Input: part model. Units: mm. Frame: model coordinates. Face numbers are marked on the shaded views. Round coordinates to 2 decimals unless told otherwise and drop trailing zeros. Order: outer loops, then holes, each group sorted by start corner. A loop starts at its lowest first (then second) coordinate and runs counter-clockwise, first axis right, second up.
Item 1: Cut plane C-C on x = -55. Output: boundary loops of the cut face in (y, z).
Item 2: Cut plane B-B on y = -3. Output: boundary loops of the cut face in (x, z).
Item 3: Mould query, pull axis X, two halves, no side actions, for the marked faces 1, 2 and 3. Classes: released by +X, released by -X, zero draft, split by the parting line, or undercut.
Item 4: Line query: L1, parallel to Z at x = 7, y = 21; L2, parallel to X at y = 21, z = -13; L3, parallel to Z at x = -53, y = 18. Output: solid intervals per line, ascending.
Item 5: First-contact query: pin 1 (12 mm diameter, centred on y = 7.5, z = -9, fed in from +X); pin 2 (3.5 mm diameter, centred on x = -7, z = -47.5, fed in from +Y); pin 3 (1.5 mm diameter, centred on y = -14.5, z = -39.5, fed in from +X); pin 4 (5 mm diameter, centred on x = -86.5, y = 11, fed in from +Z). Flat tips, straight axial feed; report the tip coordinate or a pass-through.
Item 6: Cut plane A-A on z = -30.5. Output: boundary loops of the cut face in (x, y), then the cut area to 3 significant figures.
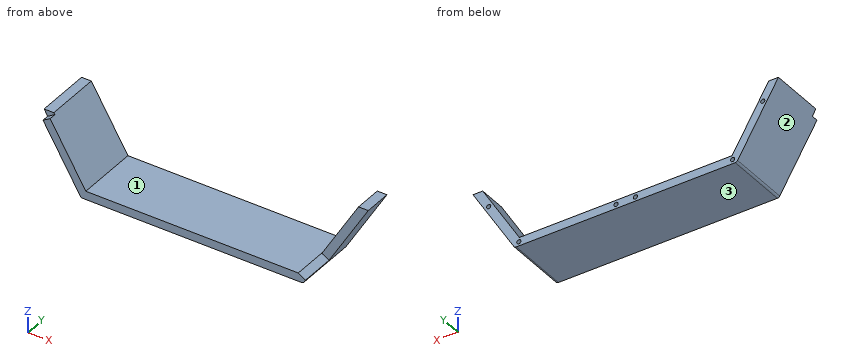
```python
from build123d import *

# Parameters (mm, degrees)
BOSS_EXTRUDE1_DEPTH = 22.5
SKETCH2_R           = 1.5
CUT_EXTRUDE1_DEPTH  = 5
FILLET1_R           = 2
SKETCH4_W           = 55
SKETCH4_H           = 25
CUT_EXTRUDE3_DEPTH  = 10
SKETCH5_W           = 5
SKETCH5_H           = 5
CUT_EXTRUDE4_DEPTH  = 10


with BuildPart() as part:
    # Sketch1 → Boss-Extrude1 (new, symmetric)
    with BuildSketch(Plane(origin=(0, 0, 0), x_dir=(1, 0, 0), z_dir=(0, 1, 0))):
        Polygon((-110, 0), (-80, 50), (80, 50), (110, 0), (103, 0), (76.6, 44), (-76.6, 44), (-103, 0), align=None)
    extrude(amount=BOSS_EXTRUDE1_DEPTH, both=True)

    # Sketch2 → Cut-Extrude1 (cut)
    with BuildSketch(Plane(origin=(0, 22.5, 0), x_dir=(1, 0, 0), z_dir=(0, 1, 0))):
        with Locations(Location((-98.701428863, 13, 0), (0, 0, 270))):
            Circle(SKETCH2_R)
        with Locations(Location((-77, 47, 0), (0, 0, 270))):
            Circle(SKETCH2_R)
        with Locations(Location((-7, 47, 0), (0, 0, 270))):
            Circle(SKETCH2_R)
        with Locations(Location((7, 47, 0), (0, 0, 90))):
            Circle(SKETCH2_R)
        with Locations(Location((77, 47, 0), (0, 0, 90))):
            Circle(SKETCH2_R)
        with Locations(Location((98.701428863, 13, 0), (0, 0, 90))):
            Circle(SKETCH2_R)
    extrude(amount=-CUT_EXTRUDE1_DEPTH, mode=Mode.SUBTRACT)

    # Fillet1
    fillet1_edges = [part.edges().sort_by_distance(p)[0] for p in [
        (-80, 0, -50),
        (80, 0, -50),
    ]]
    fillet(fillet1_edges, radius=FILLET1_R)

    # Sketch4 → Cut-Extrude3 (cut)
    with BuildSketch(Plane(origin=(80.882352941, 0, -48.529411765), x_dir=(-0.5144957554275265, 0, -0.8574929257125443), z_dir=(0.8574929257125443, 0, -0.5144957554275265))):
        with Locations((-29.094533097, -10)):
            Rectangle(SKETCH4_W, SKETCH4_H)
    extrude(amount=-CUT_EXTRUDE3_DEPTH, mode=Mode.SUBTRACT)

    # Sketch5 → Cut-Extrude4 (cut)
    with BuildSketch(Plane(origin=(-75.735294118, 0, -45.441176471), x_dir=(0.5144957554275261, 0, -0.8574929257125445), z_dir=(0.8574929257125444, 0, 0.514495755427526))):
        with Locations((-54.094533097, -20)):
            Rectangle(SKETCH5_W, SKETCH5_H)
    extrude(amount=-CUT_EXTRUDE4_DEPTH, mode=Mode.SUBTRACT)


solid = part.part
```
From the geometry:
1. outline: (-22.5, -50) - (22.5, -50) - (22.5, -44) - (-22.5, -44) - close
2. outline: (-110, 0) - (-80.58, -49.03) arc R2 ccw to (-78.87, -50) - (78.87, -50) arc R2 ccw to (80.58, -49.03) - (81.7, -47.16) - (76.43, -44) - (-76.6, -44) - (-103, 0) - close
3. face 1: undercut
3. face 2: released by -X
3. face 3: zero draft
4. L1: z = -50 to -48.5, -45.5 to -44
4. L2: x = -102.2 to -100.2, -97.2 to -95.2, 95.2 to 97.2, 100.2 to 102.2
4. L3: z = -50 to -44
5. pin 1: stops at x = 108.2
5. pin 2: stops at y = 22.5
5. pin 3: stops at x = -78.85
5. pin 4: stops at z = -23.33
6. outline: (-91.7, -22.5) - (-84.7, -22.5) - (-84.7, 22.5) - (-91.7, 22.5) - close; (84.7, 2.5) - (91.7, 2.5) - (91.7, 22.5) - (84.7, 22.5) - close
6. area: 455 mm2
